Part model, mm, in its own coordinate system. A direction names the side the tool comes from. Give positions to 0.01 mm unless a question says otherwise; leave off trailing zeros. Write each loop counter-clockwise with the first axis right and the second up, starting at its lowest first coordinate (ties: lowest second). Pieces come first, ordered by that corner, then holes. Notation, with made-up numbers: (76, -24) - (93, -24) arc R22 ccw to (93, -1) - close; hole circle Ø8 at (33, -13.75). An arc over 180 degrees is marked (long way). Answer as a JSON object with one key per item and string values. Group by question number.
```python
from build123d import *

# Parameters (mm, degrees)
F1_DEPTH = 25.4
F2_W     = 65.248069
F2_H     = 6.554596
F3_DEPTH = 10
F5_DEPTH = 10


with BuildPart() as f1:
    # F0 (on Top) → F1 (new body)
    with BuildSketch(Plane.XY):
        Polygon((35.426364, 61.360262), (-35.426364, 61.360262), (-70.852728, 0), (-35.426364, -61.360262), (35.426364, -61.360262), (70.852728, 0), align=None)
        Polygon((-55.406566, 0), (-27.703283, 47.983494), (27.703283, 47.983494), (55.406566, 0), (27.703283, -47.983494), (-27.703283, -47.983494), align=None, mode=Mode.SUBTRACT)
    extrude(amount=F1_DEPTH)

    # F2 (on face) → F3 (cut)
    with BuildSketch(Plane.XY.offset(25.4)):
        Polygon((66.450043, 1.882416), (33.826009, 58.388901), (28.149562, 55.111603), (60.773597, -1.394882), align=None)
        with Locations((1.029233, -55.211335)):
            Rectangle(F2_W, F2_H)
        Polygon((-34.855242, 56.606218), (-67.479276, 0.099733), (-61.802829, -3.177565), (-29.178795, 53.32892), align=None)
    extrude(amount=-F3_DEPTH, mode=Mode.SUBTRACT)

    # F4 (on face) → F5 (join)
    with BuildSketch(Plane(origin=(0, 0, 0), x_dir=(1, 0, 0), z_dir=(0, 0, -1))):
        Polygon((27.703283, 47.983494), (-27.703283, 47.983494), (-28.828688, 46.034235), (-55.406566, 0), (-27.703283, -47.983494), (27.703283, -47.983494), (55.406566, 0), align=None)
    extrude(amount=-F5_DEPTH)


solid = f1.part
```
1) Which spindle directions (+Z, -Z, +X, -X, +Y, -Y) get a long thin tool onto all of the face, cutting with end or side? Do faces 1 (the flat face through (53.39, 30.25, 12.52)), 2 (the flat face through (-64.681, -1.516, 20.47)). Say none if no direction does.
2) Saw through at A-A (z = 21.5). List the corners of the cut face in (x, y).
3) Drill centre lines: line 1 along X through (y, z) = (44, 24); line 2 along X through (y, z) = (53.5, 16); line 3 along X through (y, z) = (10, 16.5). Where is each one in solid material? Low to high. Write a range as from..to.
4) Saw through at C-C (y = 22.5). List the corners of the cut face in (x, z).
5) Two-plate mould, pull along X, no slides. Class faces 3 (the flat face through (52.89, -31.11, 12.52)), 4 (the flat face through (0, -61.36, 13)), 5 (the flat face through (-52.89, 31.11, 12.52)), 6 (the flat face through (-41.749, 23.656, 17.592)): +X half, -X half, draft (parallel to the pull), parting line (faces both ways), or undercut.
6) Drop flat-ended pins along their axis: P1, Ø8, axis at x = -46.5, z = 4.5, coming from the +Y side; P2, Ø6, axis at y = 7.5, z = 5, coming from the +X side; P3, Ø1, axis at x = -20, y = 41, coming from the +Z side. Give the stop position or say it passes through.
7) Saw through at D-D (z = 3.25). List the corners of the cut face in (x, y), and give its area (3 significant figures).
8) Saw through at B-B (x = -1). List the corners of the cut face in (y, z), and give its area (3 significant figures).
Checks:
{
 "1": {"face 1": "+Z, -Z, +X, +Y", "face 2": "+Z"},
 "2": {"outline": "(-70.85, 0) - (-35.43, -61.36) - (35.43, -61.36) - (70.85, 0) - (35.43, 61.36) - (-35.43, 61.36) - close; hole (-67.48, 0.1) - (-61.8, -3.18) - (-29.18, 53.33) - (-34.86, 56.61) - close; hole (-55.41, 0) - (-27.7, -47.98) - (27.7, -47.98) - (55.41, 0) - (27.7, 47.98) - (-27.7, 47.98) - close; hole (-31.59, -58.49) - (33.65, -58.49) - (33.65, -51.93) - (-31.59, -51.93) - close; hole (28.15, 55.11) - (60.77, -1.39) - (66.45, 1.88) - (33.83, 58.39) - close"},
 "3": {"line 1": "-45.45..-42.13, -34.56..-30, 30..34.56, 42.13..45.45", "line 2": "-39.96..-36.65, -29.48..29.08, 36.65..39.96", "line 3": "-65.08..-61.76, -54.19..-49.63, 49.63..54.19, 61.76..65.08"},
 "4": {"outline": "(-57.86, 0) - (57.86, 0) - (57.86, 25.4) - (54.55, 25.4) - (54.55, 15.4) - (46.98, 15.4) - (46.98, 25.4) - (42.42, 25.4) - (42.42, 10) - (-42.42, 10) - (-42.42, 25.4) - (-46.98, 25.4) - (-46.98, 15.4) - (-54.55, 15.4) - (-54.55, 25.4) - (-57.86, 25.4) - close"},
 "5": {"face 3": "+X half", "face 4": "draft", "face 5": "-X half", "face 6": "undercut"},
 "6": {"P1": "y = 49.11", "P2": "x = 68.25", "P3": "z = 10"},
 "7": {"outline": "(-70.85, 0) - (-35.43, -61.36) - (35.43, -61.36) - (70.85, 0) - (35.43, 61.36) - (-35.43, 61.36) - close", "area": "13,000 mm2"},
 "8": {"outline": "(-61.36, 0) - (61.36, 0) - (61.36, 25.4) - (47.98, 25.4) - (47.98, 10) - (-47.98, 10) - (-47.98, 25.4) - (-51.93, 25.4) - (-51.93, 15.4) - (-58.49, 15.4) - (-58.49, 25.4) - (-61.36, 25.4) - close", "area": "1,570 mm2"}
}
